from build123d import *

# Parameters (mm, degrees)
SKETCH4_R           = 52.705
BOSS_EXTRUDE1_DEPTH = 66.5988
SKETCH5_R           = 36.4109
BOSS_EXTRUDE2_DEPTH = 47.625


with BuildPart() as part:
    # Sketch1 → Revolve1 (revolve)
    with BuildSketch(Plane.XY):
        Polygon((-81.7372, -52.705), (-33.2994, -52.705), (-33.2994, -44.3484), (-81.7372, -44.6532), align=None)
        Polygon((81.7372, -44.6532), (33.2994, -44.3484), (33.2994, -52.705), (81.7372, -52.705), align=None)
    revolve(axis=Axis((-81.7372, 0, 0), (1, 0, 0)))



with BuildPart() as body_2:
    # Sketch2 → Revolve2 (revolve)
    with BuildSketch(Plane.XY):
        Polygon((30.3149, 86.4616), (30.0863, 47.625), (36.4109, 47.625), (36.4109, 86.4616), align=None)
    revolve(axis=Axis((0, 0, 0), (0, 1, 0)))


with BuildPart() as part_1:
    add(part.part)

    add(body_2.part)  # Boss-Extrude1 merges body 2
    # Sketch4 → Boss-Extrude1 (add)
    with BuildSketch(Plane(origin=(-33.2994, 0, 0), x_dir=(0, 0, -1), z_dir=(1, 0, 0))):
        Circle(SKETCH4_R)
    extrude(amount=BOSS_EXTRUDE1_DEPTH)

    # Sketch5 → Boss-Extrude2 (add)
    with BuildSketch(Plane.XZ.offset(-47.625)):
        Circle(SKETCH5_R)
    extrude(amount=BOSS_EXTRUDE2_DEPTH)

    # Sketch6 → Cut-Revolve1 (revolve, cut)
    with BuildSketch(Plane.XY):
        Polygon((-81.7372, -44.6532), (-33.2994, -44.3484), (-33.2994, -36.83), (33.2994, -36.83), (33.2994, -44.3484), (81.7372, -44.6532), (81.7372, 0), (-81.7372, 0), align=None)
    revolve(axis=Axis((81.7372, 0, 0), (-1, 0, 0)), mode=Mode.SUBTRACT)

    # Sketch7 → Cut-Revolve2 (revolve, cut)
    with BuildSketch(Plane.XY):
        Polygon((30.3149, 86.4616), (30.0863, 47.625), (24.6253, 47.625), (24.6253, 0), (0, 0), (0, 86.4616), align=None)
    revolve(axis=Axis((0, 0, 0), (0, 1, 0)), mode=Mode.SUBTRACT)


solid = part_1.part
Input: part model. Units: mm. Frame: model coordinates. Coordinates: 2 decimals unless noted, no trailing zeros. Loops run counter-clockwise (first coordinate to the right, second up) from the corner with the lowest first, then second, coordinate; pieces in that order, holes last. Notation, with made-up numbers: (-39.5, 38.25) - (9.5, 38.25) arc R30 cw to (9.5, 73.25) - close; hole circle Ø10 at (-26, 70). An arc over 180 degrees is marked (long way). Answer in a Markdown table with one row per item. Add a question column.
Item 1: Mould query, pull axis Z, two halves, no side actions, for faces 1 (the cylindrical face through (-18.15, 39.61, -16.64)), 2 (the flat face through (81.737, 43.2, -12)), 3 (the cylindrical face through (34.73, 67.99, 10.94)), 4 (the cylindrical face through (0.47, -35.13, 11.06)). Classes: released by +Z, released by -Z, zero draft, split by the parting line, or undercut.
Item 2: Section query C-C on x = 48. Return the cut outline in (y, z) (3 decimals).
Item 3: Line query: line 1 along X through (y, z) = (42.5, 0); line 2 along Z through (x, y) = (0, 42.75); line 3 along Z through (x, y) = (-3, 0) (3 decimals). Output: solid intervals per line, ascending. Write a range as [from, to].
Item 4: Contact query for flat-ended pins moving along their axis: P1, Ø8, axis at x = 37, z = 9, coming from the -Y side; P2, Ø8.5, axis at x = -7, z = 24.5, coming from the +Y side (3 decimals); P3, Ø12, axis at x = -59.5, y = 24, coming from the -Z side. Output: stop coordinate, or through.
Item 5: Section query A-A on y = 59. Return the cut outline in (x, z).
Item 6: Section query B-B on z = 9. State how many separate pieces and enclosed holes the cut face has, then the cut area to 3 significant figures.
Recorded:
| question | item | result |
|---|---|---|
| 1 | face 1 | undercut |
| 1 | face 2 | zero draft |
| 1 | face 3 | split by the parting line |
| 1 | face 4 | undercut |
| 2 | outline | circle Ø105.41 at (0, 0); hole circle Ø88.882 at (0, 0) |
| 3 | line 1 | [-33.3, -24.63], [24.63, 33.3] |
| 3 | line 2 | [-36.41, -24.63], [24.63, 36.41] |
| 3 | line 3 | [-52.705, -36.83], [36.83, 52.705] |
| 4 | P1 | y = -52.47 |
| 4 | P2 | y = 47.625 |
| 4 | P3 | z = -49.54 |
| 5 | outline | circle Ø72.82 at (0, 0); hole circle Ø60.31 at (0, 0) |
| 6 | separate pieces | 3 |
| 6 | enclosed holes | 0 |
| 6 | area | 3,430 mm^2 |
